```python
from build123d import *

# Parameters (mm, degrees)
SKETCH_1_R          = 9.52
EXTRUDE_1_DEPTH     = 2
SKETCH_4_W          = 43.1
SKETCH_4_H          = 0.98
SKETCH_4_W_2        = 46.2
SKETCH_4_H_2        = 8.602857229
EXTRUDE_2_DEPTH     = 2
SKETCH_2_R          = 2.05
CUT_EXTRUDE_1_DEPTH = 4
CUT_EXTRUDE_2_DEPTH = 10
FILLET_1_R          = 2
CUT_EXTRUDE_3_DEPTH = 2
FILLET_2_R          = 1.5


with BuildPart() as part:
    # 草图1 → 凸台-拉伸1 (new body)
    with BuildSketch(Plane.XY):
        with BuildLine():
            Line((328.542857143, -40.145714286), (-1.457142857, -40.145714286))
            ThreePointArc((-1.457142857, -40.145714286), (-41.457142857, -0.145714286), (-1.457142857, 39.854285714))
            Line((-1.457142857, 39.854285714), (328.542857143, 39.854285714))
            ThreePointArc((328.542857143, 39.854285714), (368.542857143, -0.145714286), (328.542857143, -40.145714286))
        make_face()
        with Locations((-1.457142857, -0.145714286)):
            Circle(SKETCH_1_R, mode=Mode.SUBTRACT)
        with Locations((328.542857143, -0.145714286)):
            Circle(SKETCH_1_R, mode=Mode.SUBTRACT)
        with BuildLine():
            Line((276.792857143, 35.854285714), (276.792857143, 27.854285714))
            ThreePointArc((276.792857143, 27.854285714), (275.542857143, 26.604285714), (274.292857143, 27.854285714))
            Line((274.292857143, 27.854285714), (274.292857143, 35.854285714))
            ThreePointArc((274.292857143, 35.854285714), (275.542857143, 37.104285714), (276.792857143, 35.854285714))
        make_face(mode=Mode.SUBTRACT)
        with BuildLine():
            Line((264.792857143, 27.854285714), (264.792857143, 35.854285714))
            ThreePointArc((264.792857143, 35.854285714), (266.042857143, 37.104285714), (267.292857143, 35.854285714))
            Line((267.292857143, 35.854285714), (267.292857143, 27.854285714))
            ThreePointArc((267.292857143, 27.854285714), (266.042857143, 26.604285714), (264.792857143, 27.854285714))
        make_face(mode=Mode.SUBTRACT)
    extrude(amount=EXTRUDE_1_DEPTH)

    # 草图4 → 凸台-拉伸2 (add)
    with BuildSketch(Plane.XY.offset(2)):
        with Locations((20.092857143, -40.635714286)):
            Rectangle(SKETCH_4_W, SKETCH_4_H)
        with Locations((18.542857143, 39.652857099)):
            Rectangle(SKETCH_4_W_2, SKETCH_4_H_2)
    extrude(amount=-EXTRUDE_2_DEPTH)

    # 草图2 → 切除-拉伸1 (cut)
    with BuildSketch(Plane.XY.offset(2)):
        with Locations((108.542857143, 33.854285714)):
            Circle(SKETCH_2_R)
        with Locations((198.542857143, 33.854285714)):
            Circle(SKETCH_2_R)
        with Locations((288.542857143, 33.854285714)):
            Circle(SKETCH_2_R)
        with Locations((108.542857143, -34.145714286)):
            Circle(SKETCH_2_R)
        with Locations((198.542857143, -34.145714286)):
            Circle(SKETCH_2_R)
        with Locations((288.542857143, -34.145714286)):
            Circle(SKETCH_2_R)
        with Locations((18.542857143, -34.145714286)):
            Circle(SKETCH_2_R)
        with Locations((18.542857143, 40.014285714)):
            Circle(SKETCH_2_R)
        Polygon((31.542857143, -21.145714286), (104.183898028, -21.145714286), (159.772133322, 20.854285714), (31.542857143, 20.854285714), align=None)
        Polygon((275.542857143, 20.854285714), (202.901816258, 20.854285714), (147.313580964, -21.145714286), (275.542857143, -21.145714286), align=None)
        Polygon((29.492857143, 41.064285714), (29.492857143, 38.964285714), (37.592857143, 38.964285714), (37.592857143, 41.064285714), (37.592857143, 53.579710622), (29.492857143, 53.579710622), align=None)
        Polygon((-0.507142857, 41.064285714), (-0.507142857, 38.964285714), (7.592857143, 38.964285714), (7.592857143, 41.064285714), (7.592857143, 53.579710622), (-0.507142857, 53.579710622), align=None)
    extrude(amount=-CUT_EXTRUDE_1_DEPTH, mode=Mode.SUBTRACT)

    # 草图3 → 切除-拉伸2 (cut)
    with BuildSketch(Plane.XY.offset(2)):
        with BuildLine():
            Line((183.145474057, 18.460683743), (135.97586329, -17.178577727))
            ThreePointArc((135.97586329, -17.178577727), (131.77376205, -16.593475022), (132.358864754, -12.391373783))
            Line((132.358864754, -12.391373783), (179.528475522, 23.247887686))
            ThreePointArc((179.528475522, 23.247887686), (183.730576762, 22.662784982), (183.145474057, 18.460683743))
        make_face()
    extrude(amount=-CUT_EXTRUDE_2_DEPTH, mode=Mode.SUBTRACT)

    # 圆角1
    fillet_1_edges = [part.edges().sort_by_distance(p)[0] for p in [
        (275.542857143, 20.854285714, 1),
        (275.542857143, -21.145714286, 1),
        (147.313580964, -21.145714286, 1),
        (202.901816258, 20.854285714, 1),
        (31.542857143, -21.145714286, 1),
        (31.542857143, 20.854285714, 1),
        (159.772133322, 20.854285714, 1),
        (104.183898028, -21.145714286, 1),
    ]]
    fillet(fillet_1_edges, radius=FILLET_1_R)

    # 草图5 → 切除-拉伸3 (cut)
    with BuildSketch(Plane.XY.offset(2)):
        with BuildLine():
            Line((20.806207352, -41.125714286), (29.507867411, -41.125714286))
            ThreePointArc((29.507867411, -41.125714286), (25.157037382, -37.88123609), (20.806207352, -41.125714286))
        make_face()
    extrude(amount=-CUT_EXTRUDE_3_DEPTH, mode=Mode.SUBTRACT)

    # 圆角2
    fillet_2_edges = [part.edges().sort_by_distance(p)[0] for p in [
        (37.592857143, 43.954285714, 1),
        (29.492857143, 43.954285714, 1),
        (-0.507142857, 43.954285714, 1),
        (7.592857143, 43.954285714, 1),
    ]]
    fillet(fillet_2_edges, radius=FILLET_2_R)


solid = part.part
```
Verification items for the finished model (mm, model axes). A direction names the side the tool comes from. Coordinates: 2 decimals unless noted, no trailing zeros. Loops run counter-clockwise (first coordinate to the right, second up) from the corner with the lowest first, then second, coordinate; pieces in that order, holes last. Notation, with made-up numbers: (-13, -23) -> (6, -23) arc R14 cw to (6, 3) -> close; hole circle Ø5 at (-13.75, -4). An arc over 180 degrees is marked (long way). Put each result on its own line as item: value.
1. Tool access check on faces 1 (the face through (177.572, 1.716, 1.014)), 2 (the face through (-41.385, -2.554, 0.986)). Record the directions out of +Z, -Z, +X, -X, +Y, -Y that give a thin tool (end or side, any length) a straight path to the whole face; none if there is none.
Result set:
face 1: +Z, -Z
face 2: +Z, -Z, -X
2. Section check C-C, the plane x = 170. Record the boundary of the cut face in (y, z).
Result set:
outline: (-40.15, 0) -> (-21.15, 0) -> (-21.15, 2) -> (-40.15, 2) -> close; (-4, 0) -> (8.53, 0) -> (8.53, 2) -> (-4, 2) -> close; (16.05, 0) -> (39.85, 0) -> (39.85, 2) -> (16.05, 2) -> close
3. Gauge pin test, flat ends, axial feed: P1, Ø0.6, axis at y = 30, z = 1.5, coming from the -X side; P2, Ø0.6, axis at y = 42, z = 1, coming from the +X side; P3, Ø1, axis at x = 226.5, z = 1.5, coming from the -Y side. Record the tip position at first contact, or that the pin passes through.
Result set:
P1: stops at x = -28.09
P2: stops at x = 41.64
P3: stops at y = -40.15
4. Section check A-A, the plane x = 246. Record the boundary of the cut face in (y, z).
Result set:
outline: (-40.15, 0) -> (-21.15, 0) -> (-21.15, 2) -> (-40.15, 2) -> close; (20.85, 0) -> (39.85, 0) -> (39.85, 2) -> (20.85, 2) -> close
5. Section check D-D, the plane z = 1.2. Give the number of separate pieces and of enclosed holes in the cut face, then the cut area to 3 significant figures.
Result set:
separate pieces: 1
enclosed holes: 15
area: 22,000 mm^2
6. Section check B-B, the plane y = 5.5. Record the boundary of the cut face in (x, z), then the cut area to 3 significant figures.
Result set:
outline: (-41.06, 0) -> (-9.12, 0) -> (-9.12, 2) -> (-41.06, 2) -> close; (6.21, 0) -> (31.54, 0) -> (31.54, 2) -> (6.21, 2) -> close; (139.45, 0) -> (156.04, 0) -> (156.04, 2) -> (139.45, 2) -> close; (165.99, 0) -> (182.58, 0) -> (182.58, 2) -> (165.99, 2) -> close; (275.54, 0) -> (320.88, 0) -> (320.88, 2) -> (275.54, 2) -> close; (336.21, 0) -> (368.14, 0) -> (368.14, 2) -> (336.21, 2) -> close
area: 335 mm^2
7. Mould release check, pull along Y, two halves, no side actions. Record for faces 3 (the face through (161, 11, 2)), 4 (the face through (129.51, -2.01, 1.01)), 5 (the face through (368.533, 0.734, 0.986)): pulls with the +Y half, pulls with the -Y half, needs draft (parallel to the pull), parting line crosses it, or undercut.
Result set:
face 3: needs draft
face 4: undercut
face 5: parting line crosses it
8. Thickness scan on line 1 (Y direction, x = 247.5, z = 1.7); line 2 (Y direction, x = 170, z = 0.75); line 3 (X direction, y = 35, z = 0.45). Record the ranges inside material, lowest first.
Result set:
line 1: y = -40.15 to -21.15, 20.85 to 39.85
line 2: y = -40.15 to -21.15, -4 to 8.53, 16.05 to 39.85
line 3: x = -20.56 to 106.84, 110.24 to 196.84, 200.24 to 264.79, 267.29 to 274.29, 276.79 to 286.84, 290.24 to 347.64
